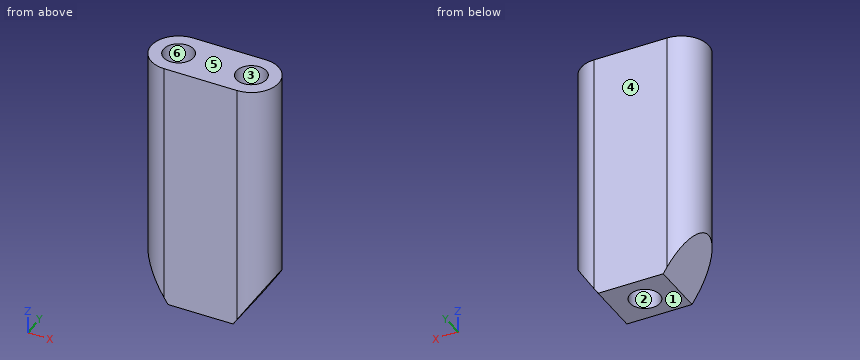
Autodesk Inventor part; units mm, degrees
ref_plane "YZ Plane" through (0, 0, 0) normal (1, 0, 0) x (0, 1, 0)
ref_plane "XZ Plane" through (0, 0, 0) normal (0, 1, 0) x (-1, 0, 0)
ref_plane "XY Plane" through (0, 0, 0) normal (0, 0, 1) x (1, 0, 0)
sketch "Sketch5" plane through (0, 0, 0) normal (0, 0, 1) x (1, 0, 0)
  line L0 (-2.8956, 2.1593) -> (2.8956, 2.1593)
  arc A0 (2.8956, -2.1593) -> (2.8956, 2.1593) centre (2.8956, 0) ccw
  line L1 (2.8956, -2.1593) -> (-2.8956, -2.1593)
  arc A1 (-2.8956, 2.1593) -> (-2.8956, -2.1593) centre (-2.8956, 0) ccw
  point P0 (0, 0)
  dimension "d44" = 2.8956
  dimension "d45" = 2.8956
extrude "Extrusion1" add sketch "Sketch5" along normal blind 20
sketch "Sketch6" plane through (0, 0, 20) normal (0, 0, 1) x (1, 0, 0)
  circle A0 centre (2.8956, 0) radius 1.1906
  circle A1 centre (-2.8956, 0) radius 1.1906
  point P0 (0, 0)
  dimension "d28" = 2.3813
  dimension "d29" = 2.8956
  dimension "d30" = 2.8956
  dimension "d31" = 2.3813
extrude "Extrusion2" cut sketch "Sketch6" against normal blind 15
sketch "Sketch7" plane through (0, 0, 0) normal (0, 0, -1) x (-1, 0, 0)
  circle A0 centre (0, 0) radius 1.1906
  dimension "d34" = 2.3813
extrude "Extrusion3" cut sketch "Sketch7" against normal blind 15
sketch "Sketch8" plane through (-2.8956, 2.1593, 0) normal (0, 1, 0) x (1, 0, 0)
  line L0 (7.9505, 0) -> (7.9505, -20)
  line L1 (7.9505, -3.81) -> (5.4781, 0)
  line L2 (0, 0) -> (5.7912, 0)
  line L3 (0.3048, 0) -> (-2.1593, -3.81)
  line L4 (-2.1593, 0) -> (-2.1593, -20)
  line L5 (5.4781, 0) -> (7.9505, 0)
  line L6 (0.3048, 0) -> (-2.1593, 0)
  line L7 (5.7912, 0) -> (0, 0)
  point P0 (2.8956, 0)
  dimension "d37" = 2.5825
  dimension "d38" = 2.5908
  dimension "d39" = 3.81
  dimension "d40" = 3.81
extrude "Extrusion4" cut sketch "Sketch8" against normal blind 15
properties part number "Splitter"
Here's how the part is built. I have some questions about the finished solid (model axes, mm). Face numbers are marked on the shaded views. A direction names the side the tool comes from. Coordinates: 2 decimals unless noted, no trailing zeros. Write each loop counter-clockwise with the first axis right and the second up, starting at its lowest first coordinate (ties: lowest second). Pieces come first, ordered by that corner, then holes. Notation, with made-up numbers: (63.5, 31.25) - (92.5, 31.25) arc R31 ccw to (92.5, 69.25) - close; hole circle Ø3 at (9.5, 39.25). An arc over 180 degrees is marked (long way). Use one line per item in the form item = value.
1) Thinking about a two-plate mould opening in Y: for the marked faces 3, 4, 5 and 6, which applies, released by +Y, released by -Y, zero draft, split by the parting line, or undercut?
Solved:
face_3 = undercut
face_4 = released by +Y
face_5 = zero draft
face_6 = undercut
2) Suppose I cut it at B-B, the plane x = 0. Write out the boundary of the cut face in (y, z), plus the area to 3 significant figures.
Solved:
outline = (-2.16, 0) - (-1.19, 0) - (-1.19, 15) - (1.19, 15) - (1.19, 0) - (2.16, 0) - (2.16, 20) - (-2.16, 20) - close
area = 50.7 mm2
3) I'm going to push flat-ended pins straight in: P1, Ø2, axis at x = -4, z = 11, coming from the -Y side; P2, Ø1.5, axis at y = -1.5, z = 9, coming from the +X side. Where does each tip first touch, or does it pass through?
Solved:
P1 = -2.16
P2 = 4.92
4) Suppose I cut it at A-A, the plane z = 14.75. Write out the boundary of the cut face in (x, y) (3 decimals), plus the area to 3 significant figures.
Solved:
outline = (-2.896, -2.159) - (2.896, -2.159) arc R2.159 ccw to (2.896, 2.159) - (-2.896, 2.159) arc R2.159 ccw to start; hole circle Ø2.381 at (-2.896, 0); hole circle Ø2.381 at (0, 0); hole circle Ø2.381 at (2.896, 0)
area = 26.3 mm2
5) On a 3-axis mill with a long thin cutter (end or side, diameter ignored), from which of +Z, -Z, +X, -X, +Y, -Y can I reach the whole of each face in a straight line? I mean the marked faces 1 and 2. Say none if no direction works.
Solved:
face_1 = -Z, +X, -X, +Y, -Y
face_2 = -Z
6) Suppose I cut it at D-D, the plane y = 0. Write out the boundary of the cut face in (x, z) (1 decimal).
Solved:
outline = (-5.1, 3.8) - (-2.6, 0) - (-1.2, 0) - (-1.2, 15) - (1.2, 15) - (1.2, 0) - (2.6, 0) - (5.1, 3.8) - (5.1, 20) - (4.1, 20) - (4.1, 5) - (1.7, 5) - (1.7, 20) - (-1.7, 20) - (-1.7, 5) - (-4.1, 5) - (-4.1, 20) - (-5.1, 20) - close
7) Suppose I cut it at C-C, the plane z = 17. Write out the boundary of the cut face in (x, y) (3 decimals).
Solved:
outline = (-2.896, -2.159) - (2.896, -2.159) arc R2.159 ccw to (2.896, 2.159) - (-2.896, 2.159) arc R2.159 ccw to start; hole circle Ø2.381 at (-2.896, 0); hole circle Ø2.381 at (2.896, 0)
8) I need wall thicknesses on line 1 (X direction, y = 0.85, z = 8); line 2 (X direction, y = -0.7, z = 14.5); line 3 (X direction, y = -0.7, z = 18). Which ranges of each line are inside material? Lowest first, please.
Solved:
line_1 = -4.88 to -3.73, -2.06 to -0.83, 0.83 to 2.06, 3.73 to 4.88
line_2 = -4.94 to -3.86, -1.93 to -0.96, 0.96 to 1.93, 3.86 to 4.94
line_3 = -4.94 to -3.86, -1.93 to 1.93, 3.86 to 4.94
